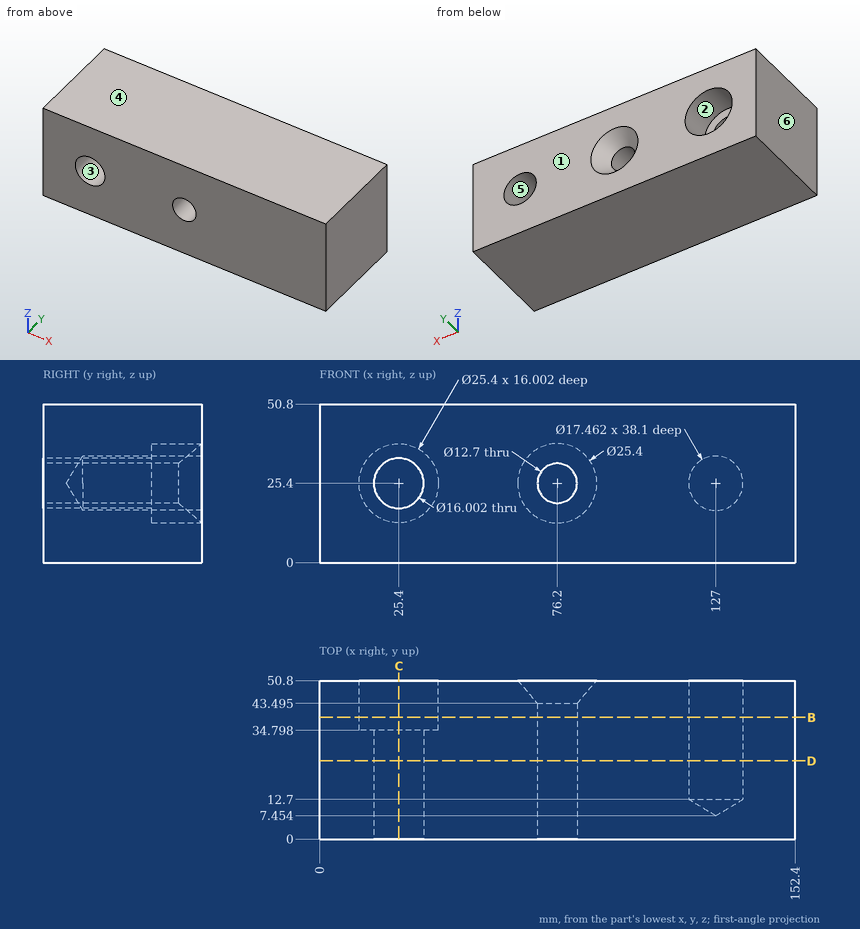
Source: three-view drawing plus pictorial views. Frame: mm from the lowest corner of the part. A direction names the side the tool comes from. Round coordinates to 2 decimals unless told otherwise and drop trailing zeros. Order: outer loops, then holes, each group sorted by start corner. A loop starts at its lowest first (then second) coordinate and runs counter-clockwise, first axis right, second up. Notation, with made-up numbers: (80, 53) - (135, 53) arc R23 cw to (135, 61) - close; hole circle Ø9 at (17.5, 1.25). An arc over 180 degrees is marked (long way). Answer in a Markdown table with one row per item.
Item 1: Reachability of the marked faces 1 and 2 from +Z, -Z, +X, -X, +Y, -Y: full face, straight path, thin tool, end or side. Return the list, or none.
Model answer:
| item | result |
|---|---|
| face 1 | +Z, -Z, +X, -X, +Y |
| face 2 | +Y |
Item 2: Section query D-D (y = 25). Return the cut outline in (x, z).
Model answer:
| item | result |
|---|---|
| outline | (0, 0) - (152.4, 0) - (152.4, 50.8) - (0, 50.8) - close; hole circle Ø16 at (25.4, 25.4); hole circle Ø12.7 at (76.2, 25.4); hole circle Ø17.46 at (127, 25.4) |
Item 3: Section query C-C (x = 25.4). Return the cut outline in (y, z), then the cut area to 3 significant figures.
Model answer:
| item | result |
|---|---|
| outline | (0, 0) - (50.8, 0) - (50.8, 12.7) - (34.8, 12.7) - (34.8, 17.4) - (0, 17.4) - close; (0, 33.4) - (34.8, 33.4) - (34.8, 38.1) - (50.8, 38.1) - (50.8, 50.8) - (0, 50.8) - close |
| area | 1,620 mm² |
Item 4: Mould query, pull axis X, two halves, no side actions, for the marked faces 3, 4, 5 and 6. Classes: released by +X, released by -X, zero draft, split by the parting line, or undercut.
Model answer:
| item | result |
|---|---|
| face 3 | undercut |
| face 4 | zero draft |
| face 5 | undercut |
| face 6 | released by -X |
Item 5: Pin query (flat end, axial travel): pin 1 (10 mm diameter, centred on x = 75, z = 31.5, fed in from +Y) (1 decimal); pin 2 (12.5 mm diameter, centred on x = 22, z = 21.5, fed in from +Y); pin 3 (10 mm diameter, centred on x = 76.2, z = 25.4, fed in from +Y). Return the tip coordinate at first contact, or that it passes through.
Model answer:
| item | result |
|---|---|
| pin 1 | stops at y = 49.1 |
| pin 2 | stops at y = 34.8 |
| pin 3 | passes through |
Item 6: Section query B-B (y = 39). Return the cut outline in (x, z).
Model answer:
| item | result |
|---|---|
| outline | (0, 0) - (152.4, 0) - (152.4, 50.8) - (0, 50.8) - close; hole circle Ø25.4 at (25.4, 25.4); hole circle Ø12.7 at (76.2, 25.4); hole circle Ø17.46 at (127, 25.4) |
Item 7: Line query: line 1 (X direction, y = 27, z = 25); line 2 (Z direction, x = 25.4, y = 47.75); line 3 (Z direction, x = 76, y = 16). Output: solid intervals per line, ascending.
Model answer:
| item | result |
|---|---|
| line 1 | x = 0 to 17.41, 33.39 to 69.86, 82.54 to 118.28, 135.72 to 152.4 |
| line 2 | z = 0 to 12.7, 38.1 to 50.8 |
| line 3 | z = 0 to 19.05, 31.75 to 50.8 |
